Read the model definition and answer for the solid it produces. Units are mm, in the model's axes. Coordinates: 2 decimals unless noted, no trailing zeros. Use CSV: the item, a comma, the result in double quotes.
from build123d import *

# Parameters (mm, degrees)
SWEEP1_PROFILE_R = 0.75


with BuildPart() as part:
    # Sweep1: sweep along a curve in space
    with BuildLine() as sweep1_path:
        Line((-96.760776121, -3.47025774, 78.252711823), (-78.084348541, -0.522963163, 86.961878631))
        ThreePointArc((-96.760776121, -3.47025774, 78.252711823), (-99.112397911, -4.596881054, 76.226314182), (-99.548244883, -6.60263734, 73.639294338))
        Line((-99.548244883, -6.60263734, 73.639294338), (-99.328473076, -7.317696757, 72.819094788))
        ThreePointArc((-98.82832928, -8.022963163, 70.95253273), (-99.09453566, -7.841136399, 71.946028463), (-99.328473076, -7.317696757, 72.819094788))
        Line((-98.627122104, -8.022963163, 70.201617327), (-98.82832928, -8.022963163, 70.95253273))
        ThreePointArc((-98.627122104, -8.022963163, 70.201617327), (-98.353918152, -7.831121447, 69.182006297), (-98.115655477, -7.280131794, 68.292797886))
        Line((-98.115655477, -7.280131794, 68.292797886), (-97.882684409, -6.49206537, 67.423338024))
        ThreePointArc((-93.143377561, -3.311786612, 64.859921351), (-96.209258102, -4.441131936, 65.426107931), (-97.882684409, -6.49206537, 67.423338024))
        Line((-93.143377561, -3.311786612, 64.859921351), (-72.649148593, -0.522963163, 66.677436279))
    # Sweep1 profile (on start of the path) → Sweep1 (sweep)
    with BuildSketch(Plane(origin=(-72.649148593, -0.522963163, 66.677436279), x_dir=(0.13483580164041467, -0.9908679561858819, 0), z_dir=(-0.9870642774001727, -0.1343182028271198, -0.08753703598916203))):
        Circle(SWEEP1_PROFILE_R)
    sweep(path=sweep1_path.line)


solid = part.part
1. For a pull along Z with two mould halves and no side action, classify faces 1 (the flat face through (-72.651, -0.513, 66.688)), 2 (the cylindrical face through (-83.117, -1.849, 66.497)) as pulls with the +Z half, pulls with the -Z half, needs draft (parallel to the pull), parting line crosses it, or undercut.
Solutions:
face 1,"pulls with the +Z half"
face 2,"undercut"
2. Each of these flat-tipped pins is pushed along its axis until it touches: pin 1 Ø8 at (x, z) = (-76.5, 83) entering from +Y; pin 2 Ø10 at (x, z) = (-93, 70.5) entering from +Y; pin 3 Ø4 at (y, z) = (-3, 77) entering from +X. Where does it stop, or does it pass through?
Solutions:
pin 1,"stops at y = 0.17"
pin 2,"stops at y = -2.75"
pin 3,"stops at x = -93.38"
3. Find the intervals of material crossed by line 1 along Z through (x, y) = (-97.5, -6.75); line 2 along Z through (x, y) = (-85.25, -2.5); line 3 along Y through (x, z) = (-78.25, 86.75), in increasing order.
Solutions:
line 1,"z = 66.68 to 68.45"
line 2,"z = 64.85 to 66.26"
line 3,"y = -1.3 to 0.19"
